from build123d import *

# Parameters (mm, degrees)
SKETCH1_W           = 186
SKETCH1_H           = 196
BOSS_EXTRUDE1_DEPTH = 3
BOSS_EXTRUDE2_START = -53.4
BOSS_EXTRUDE2_DEPTH = 50.4
CHAMFER1_SIZE       = 10
SKETCH1_4_W         = 5
SKETCH1_4_H         = 0.8
SKETCH1_4_H_2       = 15
BOSS_EXTRUDE3_DEPTH = 42.9
CHAMFER2_SIZE       = 2.5
SKETCH2_R           = 2.35
SKETCH2_R_2         = 1.8
CUT_EXTRUDE2_DEPTH  = 4.5
SKETCH2_3_R         = 1.8
CUT_EXTRUDE3_DEPTH  = 8
FILLET1_R           = 7
FILLET2_R           = 4


with BuildPart() as part:
    # Sketch1 → Boss-Extrude1 (new body)
    with BuildSketch(Plane(origin=(0, 0, 0), x_dir=(1, 0, 0), z_dir=(0, 1, 0))):
        with Locations((93, 98)):
            Rectangle(SKETCH1_W, SKETCH1_H)
    extrude(amount=-BOSS_EXTRUDE1_DEPTH)

    # Sketch1<3> → Boss-Extrude2 (add)
    with BuildSketch(Plane(origin=(0, 0, 0), x_dir=(1, 0, 0), z_dir=(0, 1, 0)).offset(BOSS_EXTRUDE2_START)):
        Polygon((186, 196), (158.2, 196), (158.2, 191), (181, 191), (181, 55.55), (186, 55.55), align=None)
        Polygon((81.6, 191), (81.6, 196), (0, 196), (0, 0), (186, 0), (186, 38.95), (181, 38.95), (181, 5), (5, 5), (5, 191), align=None)
    extrude(amount=BOSS_EXTRUDE2_DEPTH)

    # Chamfer1
    chamfer1_edges = [part.edges().sort_by_distance(p)[0] for p in [
        (5, -28.2, -191),
        (5, -28.2, -5),
        (181, -28.2, -5),
        (181, -28.2, -191),
    ]]
    chamfer(chamfer1_edges, length=CHAMFER1_SIZE)

    # Sketch1<4> → Boss-Extrude3 (add)
    with BuildSketch(Plane(origin=(0, 0, 0), x_dir=(1, 0, 0), z_dir=(0, 1, 0))):
        with Locations((183.5, 55.15)):
            Rectangle(SKETCH1_4_W, SKETCH1_4_H)
        with Locations((183.5, 47.25)):
            Rectangle(SKETCH1_4_W, SKETCH1_4_H_2)
        with Locations((183.5, 39.35)):
            Rectangle(SKETCH1_4_W, SKETCH1_4_H)
    extrude(amount=-BOSS_EXTRUDE3_DEPTH)

    # Chamfer2
    chamfer2_edges = [part.edges().sort_by_distance(p)[0] for p in [
        (183.5, -42.9, -55.55),
        (183.5, -42.9, -38.95),
    ]]
    chamfer(chamfer2_edges, length=CHAMFER2_SIZE)

    # Sketch2 → Cut-Extrude2 (cut)
    # profile 1 of 4: a face of its own
    with BuildSketch(Plane.XZ.offset(53.4)):
        with Locations(Location((6.5, -6.5, 0), (0, 0, 270))):
            Circle(SKETCH2_R)
        with Locations(Location((6.5, -6.5, 0), (0, 0, 270))):
            Circle(SKETCH2_R_2, mode=Mode.SUBTRACT)
    # profile 2 of 4: a face of its own
    with BuildSketch(Plane.XZ.offset(53.4)):
        with Locations(Location((179.5, -6.5, 0), (0, 0, 90))):
            Circle(SKETCH2_R)
        with Locations(Location((179.5, -6.5, 0), (0, 0, 90))):
            Circle(SKETCH2_R_2, mode=Mode.SUBTRACT)
    # profile 3 of 4: a face of its own
    with BuildSketch(Plane.XZ.offset(53.4)):
        with Locations(Location((179.5, -189.5, 0), (0, 0, 270))):
            Circle(SKETCH2_R)
        with Locations(Location((179.5, -189.5, 0), (0, 0, 270))):
            Circle(SKETCH2_R_2, mode=Mode.SUBTRACT)
    # profile 4 of 4: a face of its own
    with BuildSketch(Plane.XZ.offset(53.4)):
        with Locations(Location((6.5, -189.5, 0), (0, 0, 90))):
            Circle(SKETCH2_R)
        with Locations(Location((6.5, -189.5, 0), (0, 0, 90))):
            Circle(SKETCH2_R_2, mode=Mode.SUBTRACT)
    extrude(amount=-CUT_EXTRUDE2_DEPTH, mode=Mode.SUBTRACT)

    # Sketch2<3> → Cut-Extrude3 (cut)
    with BuildSketch(Plane.XZ.offset(53.4)):
        with Locations(Location((6.5, -6.5, 0), (0, 0, 270))):
            Circle(SKETCH2_3_R)
        with Locations(Location((6.5, -189.5, 0), (0, 0, 270))):
            Circle(SKETCH2_3_R)
        with Locations(Location((179.5, -189.5, 0), (0, 0, 270))):
            Circle(SKETCH2_3_R)
        with Locations(Location((179.5, -6.5, 0), (0, 0, 90))):
            Circle(SKETCH2_3_R)
    extrude(amount=-CUT_EXTRUDE3_DEPTH, mode=Mode.SUBTRACT)

    # Fillet1
    fillet1_edges = [part.edges().sort_by_distance(p)[0] for p in [
        (0, -26.7, 0),
        (186, -26.7, 0),
        (186, -26.7, -196),
        (0, -26.7, -196),
    ]]
    fillet(fillet1_edges, radius=FILLET1_R)

    # Fillet2
    # the kernel refuses this fillet: 4 mm, written as the material it takes off along each edge
    with BuildSketch(Plane(origin=(179, 0, -7), x_dir=(0, 0, 1), z_dir=(-1, 0, 0))) as fillet2_piece_1:
        with BuildLine():
            CenterArc((7 - FILLET2_R, -FILLET2_R), FILLET2_R, 0, 90)
            Line((7, -FILLET2_R), (7, 0))
            Line((7, 0), (7 - FILLET2_R, 0))
        make_face()
    revolve(axis=Axis((179, 0, -7), (0, 1, 0)), revolution_arc=90, mode=Mode.SUBTRACT)
    with BuildSketch(Plane(origin=(7, 0, 0), x_dir=(0, 0, -1), z_dir=(1, 0, 0))) as fillet2_piece_2:
        with BuildLine():
            CenterArc((FILLET2_R, -FILLET2_R), FILLET2_R, 90, 90)
            Line((0, -FILLET2_R), (0, 0))
            Line((0, 0), (FILLET2_R, 0))
        make_face()
    extrude(amount=172, mode=Mode.SUBTRACT)
    with BuildSketch(Plane(origin=(7, 0, -7), x_dir=(0, 0, 1), z_dir=(1, 0, 0))) as fillet2_piece_3:
        with BuildLine():
            CenterArc((7 - FILLET2_R, FILLET2_R), FILLET2_R, 270, 90)
            Line((7, FILLET2_R), (7, 0))
            Line((7, 0), (7 - FILLET2_R, 0))
        make_face()
    revolve(axis=Axis((7, 0, -7), (0, -1, 0)), revolution_arc=90, mode=Mode.SUBTRACT)
    with BuildSketch(Plane(origin=(0, 0, -189), x_dir=(1, 0, 0), z_dir=(0, 0, 1))) as fillet2_piece_4:
        with BuildLine():
            CenterArc((FILLET2_R, -FILLET2_R), FILLET2_R, 90, 90)
            Line((0, -FILLET2_R), (0, 0))
            Line((0, 0), (FILLET2_R, 0))
        make_face()
    extrude(amount=182, mode=Mode.SUBTRACT)
    with BuildSketch(Plane(origin=(7, 0, -189), x_dir=(0, 0, -1), z_dir=(1, 0, 0))) as fillet2_piece_5:
        with BuildLine():
            CenterArc((7 - FILLET2_R, -FILLET2_R), FILLET2_R, 0, 90)
            Line((7, -FILLET2_R), (7, 0))
            Line((7, 0), (7 - FILLET2_R, 0))
        make_face()
    revolve(axis=Axis((7, 0, -189), (0, 1, 0)), revolution_arc=90, mode=Mode.SUBTRACT)
    with BuildSketch(Plane(origin=(179, 0, -196), x_dir=(0, -1, 0), z_dir=(-1, 0, 0))) as fillet2_piece_6:
        with BuildLine():
            CenterArc((FILLET2_R, FILLET2_R), FILLET2_R, 180, 90)
            Line((0, FILLET2_R), (0, 0))
            Line((0, 0), (FILLET2_R, 0))
        make_face()
    extrude(amount=172, mode=Mode.SUBTRACT)
    with BuildSketch(Plane(origin=(179, 0, -189), x_dir=(0, 0, -1), z_dir=(-1, 0, 0))) as fillet2_piece_7:
        with BuildLine():
            CenterArc((7 - FILLET2_R, FILLET2_R), FILLET2_R, 270, 90)
            Line((7 - FILLET2_R, 0), (7, 0))
            Line((7, 0), (7, FILLET2_R))
        make_face()
    revolve(axis=Axis((179, 0, -189), (0, -1, 0)), revolution_arc=90, mode=Mode.SUBTRACT)
    with BuildSketch(Plane(origin=(186, 0, -189), x_dir=(-1, 0, 0), z_dir=(0, 0, 1))) as fillet2_piece_8:
        with BuildLine():
            CenterArc((FILLET2_R, FILLET2_R), FILLET2_R, 180, 90)
            Line((0, FILLET2_R), (0, 0))
            Line((0, 0), (FILLET2_R, 0))
        make_face()
    extrude(amount=182, mode=Mode.SUBTRACT)


solid = part.part
CAD build for the part. Positions are in the model's coordinates, mm. A direction names the side the tool comes from. Round coordinates to 2 decimals unless told otherwise and drop trailing zeros. Loops run counter-clockwise (first coordinate to the right, second up) from the corner with the lowest first, then second, coordinate; pieces in that order, holes last. Notation, with made-up numbers: M -13.5,-31.5 L -5.5,-31.5 A32 cw -5.5,3.5 Z; hole C 47,-38.75 d11. An arc over 180 degrees is marked long. One line per question, with ' | ' between items. Start each with the question number.
Item 1: Cut at D-D, the plane x = 29.5. Write the cut outline in (y, z), plus the area to 3 significant figures.
Item 2: Cut at B-B, the plane z = -183.5. Write the cut outline in (x, y).
Item 3: Two-plate mould, pull along X, no slides. Class faces 1 (the cylindrical face through (177.415, -51.182, -190.584)), 2 (the flat face through (183, -49, -55.55)), 3 (the cylindrical face through (4.415, -51.182, -7.584)), 4 (the cylindrical face through (2, -28.4, -2.1)): pulls with the +X half, pulls with the -X half, needs draft (parallel to the pull), parting line crosses it, or undercut.
Item 4: Which spindle directions (+Z, -Z, +X, -X, +Y, -Y) get a long thin tool onto all of the face, cutting with end or side? Do faces 5 (the flat face through (10, -29, -186)), 6 (the flat face through (158.2, -29, -194)), 7 (the cylindrical face through (184, -29, -2.1)), 8 (the flat face through (183, -42.9, -47)). Say none if no direction does.
Item 5: Wall check: line 1 (X direction, y = -46.5, z = -189.5); line 2 (X direction, y = -45, z = -26.5); line 3 (X direction, y = -50, z = -189). Give the ranges that are in metal, low to high.
Item 6: Cut at C-C, the plane y = -15. Write the cut outline in (x, z), plus the area to 3 significant figures.
Item 7: Pin check, flat tips, straight feed: pin 1 Ø4.5 at (x, z) = (6.5, -189.5) entering from +Y; pin 2 Ø3 at (x, z) = (179.5, -6.5) entering from -Y; pin 3 Ø5.5 at (x, y) = (183, -50.5) entering from +Z; pin 4 Ø6 at (x, z) = (116, -116) entering from -Y. Stop position of each tip, or through.
Item 8: Cut at A-A, the plane x = 104.5. Write the cut outline in (y, z).
Responses:
1) outline: M -53.4,-196 L -4,-196 A4 ccw 0,-192 L 0,-4 A4 ccw -4,0 L -53.4,0 L -53.4,-5 L -3,-5 L -3,-191 L -53.4,-191 Z | area: 1,090 mm²
2) outline: M 0,-53.4 L 7.5,-53.4 L 7.5,-3 L 178.5,-3 L 178.5,-53.4 L 186,-53.4 L 186,-4 A4 ccw 182,0 L 4,0 A4 ccw 0,-4 Z
3) face 1: undercut | face 2: needs draft | face 3: undercut | face 4: pulls with the -X half
4) face 5: -Y | face 6: -Z, -Y | face 7: +Z, +X, +Y, -Y | face 8: +X, -Y
5) line 1: x = 0.02 to 4.7, 8.3 to 13.5, 172.5 to 177.7, 181.3 to 185.98 | line 2: x = 0 to 5, 181 to 186 | line 3: x = 0 to 4.2, 8.8 to 13, 173 to 177.2, 181.8 to 186
6) outline: M 0,-189 A7 ccw 7,-196 L 81.6,-196 L 81.6,-191 L 15,-191 L 5,-181 L 5,-15 L 15,-5 L 171,-5 L 181,-15 L 181,-181 L 171,-191 L 158.2,-191 L 158.2,-196 L 179,-196 A7 ccw 186,-189 L 186,-7 A7 ccw 179,0 L 7,0 A7 ccw 0,-7 Z | area: 3,490 mm²
7) pin 1: stops at y = 0 | pin 2: stops at y = -45.4 | pin 3: stops at z = -0.11 | pin 4: stops at y = -3
8) outline: M -53.4,-5 L -3,-5 L -3,-195.87 A4 ccw 0,-192 L 0,-4 A4 ccw -4,0 L -53.4,0 Z
